Input: part model. Units: mm. Frame: model coordinates. Coordinates: 2 decimals unless noted, no trailing zeros. Loops run counter-clockwise (first coordinate to the right, second up) from the corner with the lowest first, then second, coordinate; pieces in that order, holes last.
(1) Section A-A, the plane z = 20.75. Return loops of the section in (x, y), then the cut area to 3 significant figures.
(2) Section B-B, the plane z = 4.25. Return loops of the section in (x, y).
(3) Mould query, pull axis Y, two halves, no side actions, for faces 1 (the face through (2.13, 2.24, 6.08)), 2 (the face through (2.13, 12.88, 6.08)), 3 (the face through (3.4, 11.6, 7)). Classes: released by +Y, released by -Y, zero draft, split by the parting line, or undercut.
(4) Section C-C, the plane x = 21. Return loops of the section in (y, z), then the cut area to 3 significant figures.
(5) Section D-D, the plane x = 29. Return loops of the section in (y, z), then the cut area to 3 significant figures.
(6) Line query: L1, parallel to Y at x = 21, z = 4.25; L2, parallel to X at y = 0.75, z = 24; L3, parallel to X at y = 4.25, z = 6. Output: solid intervals per line, ascending.
(7) Contact query for flat-ended pins moving along their axis: P1, Ø1.3, axis at x = 42, y = 13.5, coming from the -Z side; P2, Ø3, axis at x = 27, y = 8.5, coming from the +Z side; P3, Ø4, axis at x = 10.5, y = 9.5, coming from the -Z side. Output: stop coordinate, or through.
```python
from build123d import *

# Parameters (mm, degrees)
F1_DEPTH  = 12
F3_DEPTH  = 25
F4_T      = -1.8
F5_R      = 5.7
F6_R      = 7.5
F8_R      = 3
F9_DEPTH  = 16.37
F10_R     = 1.2
F11_DEPTH = 16.3887303416
F14_DEPTH = 13.87
F17_DEPTH = 9.8
F19_DEPTH = 9.8


with BuildPart() as f1:
    # F0 (on Top) → F1 (new body)
    with BuildSketch(Plane.XY):
        Polygon((0, 15.12), (0, 0), (42.3, -0.125), (42.3, 15.245), align=None)
    extrude(amount=F1_DEPTH)

    # F2 (on face) → F3 (cut)
    with BuildSketch(Plane(origin=(0, 0, 0), x_dir=(0.9999956338, -0.0029550698, 0), z_dir=(-0.0029550698, -0.9999956338, 0))):
        Polygon((42.3001846923, 0), (42.3001846923, 9.2), (19.6, 0), align=None)
        with BuildLine():
            Line((0, 0), (19.6, 0))
            ThreePointArc((19.6, 0), (9.8, 1.15), (0, 0))
        make_face()
    extrude(amount=-F3_DEPTH, mode=Mode.SUBTRACT)

    # F4
    f4_openings = [f1.faces().sort_by_distance(p)[0] for p in [
        (21.207806, 7.56, 12),
    ]]
    offset(amount=F4_T, openings=f4_openings)

    # F5
    f5_edges = [f1.edges().sort_by_distance(p)[0] for p in [
        (1.8, 13.325311, 7.10578),
        (1.8, 1.794689, 7.108929),
    ]]
    fillet(f5_edges, radius=F5_R)

    # F6#2 (call 1 of 2: OpenCascade refuses the feature's edges together)
    f6_2_edges = [f1.edges().sort_by_distance(p)[0] for p in [
        (0, 0, 6),
    ]]
    fillet(f6_2_edges, radius=F6_R)

    # F6 (call 2 of 2)
    f6_edges = [f1.edges().sort_by_distance(p)[0] for p in [
        (0, 15.12, 6),
    ]]
    fillet(f6_edges, radius=F6_R)

    # F8 (on offset) → F9 (join)
    with BuildSketch(Plane(origin=(-0.0014775349, -0.4999978169, 0), x_dir=(0.9999956338, -0.0029550698, 0), z_dir=(-0.0029550698, -0.9999956338, 0))):
        with Locations((39.3001846923, 12)):
            Circle(F8_R)
    extrude(amount=-F9_DEPTH)

    # F10 (on face) → F11 (cut, through all)
    with BuildSketch(Plane(origin=(-0.0014775349, -0.4999978169, 0), x_dir=(0.9999956338, -0.0029550698, 0), z_dir=(-0.0029550698, -0.9999956338, 0))):
        with Locations((39.3001846923, 12)):
            Circle(F10_R)
    extrude(amount=-F11_DEPTH, mode=Mode.SUBTRACT)

    # F13 (on offset) → F14 (join)
    with BuildSketch(Plane(origin=(-0.0424641585, 14.3698712402, 0), x_dir=(-0.9999956338, -0.0029550698, 0), z_dir=(-0.0029550698, 0.9999956338, 0))):
        Polygon((-39.6163160442, 9.2177886928), (-28.3448653482, 5.1912576891), (-28.3448653482, 12), (-33.3448653482, 12), (-37.8970582696, 15), (-37.8970582696, 21.4), (-34.1948653482, 22.55), (-34.1948653482, 24.9), (-42.9948653482, 24.9), (-42.9948653482, 21.7), (-41.8448653482, 21.7), (-41.8448653482, 13.4442944811), (-36.9448653482, 13.4442944811), align=None)
    extrude(amount=-F14_DEPTH)

    # F16 (on offset) → F17 (cut)
    with BuildSketch(Plane(origin=(0.0082741956, 2.7999877746, 0), x_dir=(-0.9999956338, 0.0029550698, 0), z_dir=(0.0029550698, 0.9999956338, 0))):
        Polygon((-45.8104334942, 12.5648554603), (-19.4509569667, 1.8818065187), (-19.4509569667, 29.0965877719), (-45.8104334942, 29.0965877719), align=None)
    extrude(amount=F17_DEPTH, mode=Mode.SUBTRACT)

    # F18 (on face) → F19 (join, through all)
    with BuildSketch(Plane(origin=(0.0082741956, 2.7999877746, 0), x_dir=(-0.9999956338, 0.0029550698, 0), z_dir=(0.0029550698, 0.9999956338, 0))):
        Polygon((-42.3346940311, 15.5157536155), (-42.2919104606, 11.1388577274), (-40.7162009106, 10.5002493611), (-40.7162009106, 13.6316680383), align=None)
    extrude(amount=F19_DEPTH)


solid = f1.part
```
Report:
1. outline: (37.85, 14.48) - (37.86, 12.49) - (41.81, 12.48) - (41.8, 14.49) - close; (37.89, 2.69) - (37.9, 0.61) - (41.84, 0.62) - (41.84, 2.68) - close
1. area: 16.1 mm2
2. outline: (0, 7.48) arc R7.5 ccw to (7.48, -0.02) - (30.09, -0.09) - (30.13, 15.21) - (7.48, 15.14) arc R7.5 ccw to (0, 7.64) - close; hole (1.8, 7.48) arc R5.7 ccw to (7.48, 1.78) - (25.3, 1.73) - (25.33, 13.39) - (7.48, 13.34) arc R5.7 ccw to (1.8, 7.64) - close
3. face 1: released by -Y
3. face 2: released by +Y
3. face 3: undercut
4. outline: (-0.06, 0.57) - (15.18, 0.55) - (15.18, 12) - (13.38, 12) - (13.38, 2.49) - (1.74, 2.51) - (1.74, 12) - (-0.06, 12) - close
4. area: 63.8 mm2
5. outline: (-0.09, 3.81) - (15.21, 3.79) - (15.21, 12) - (12.51, 12) - (12.51, 5.74) - (2.71, 5.75) - (2.71, 12) - (-0.09, 12) - close
5. area: 64.1 mm2
6. L1: y = -0.06 to 1.74, 13.38 to 15.18
6. L2: x = 34.19 to 42.99
6. L3: x = 0.73 to 2.8, 29.62 to 34.42
7. P1: stops at z = 8.8
7. P2: stops at z = 5.54
7. P3: stops at z = 1.07
